Could you check a few things on this model? Use its own coordinates, in mm. A direction names the side the tool comes from. Round coordinates to 2 decimals unless told otherwise and drop trailing zeros. Write each loop counter-clockwise with the first axis right and the second up, starting at its lowest first coordinate (ties: lowest second). Pieces come first, ordered by that corner, then holes. Notation, with made-up numbers: (42.25, 5.5) -> (55.25, 5.5) arc R24 ccw to (55.25, 17.5) -> close; hole circle Ø2 at (62, -8). An arc over 180 degrees is marked (long way). Answer as CSV lines item,"result". Start each with the question number.
Q1. Imagine slicing it at B-B on x = -0.75. Please give me the cut outline in (y, z).
Q2. Imagine slicing it at A-A on z = 30. Please give me the cut outline in (x, y), and give its area (3 significant figures).
Q3. Imagine slicing it at D-D on y = -2.25. Please give me the cut outline in (x, z).
Q4. For faces 4 (the flat face through (-6, -3.355, 11)), 5 (the flat face through (3, 3, 50)), 6 (the flat face through (-2, -6, 41)), which set-ups out of +Z, -Z, +X, -X, +Y, -Y let a thin tool reach every point of the face, with its end or its side?
Q5. If we mould it in two halves opening along Z, with no side actions, what happens to faces 1 (the flat face through (3, 3, -20)), 2 (the flat face through (-3.974, 4.075, 43.535)), 3 (the flat face through (-1, 7.895, 15))? For each: pulls with the +Z half, pulls with the -Z half, needs draft (parallel to the pull), parting line crosses it, or undercut.
Q6. If I drill on line 1 (Z direction, x = -0.75, y = 5.15); line 2 (Y direction, x = -5.75, z = 38.5); line 3 (X direction, y = -1.25, z = 13.5), over which ranges is the centre line in solid material (lowest first)? Write a range as [from, to].
Q7. Will this pin go through, and if not, where does the flat tip stop? pin 1 Ø4 at (x, z) = (-0.75, 30) entering from +Y.
Q8. Imagine slicing it at C-C on z = -7.5. Please give me the cut outline in (x, y).
from build123d import *
from build123d.topology import SkipClean

# Parameters (mm, degrees)
BOSS_EXTRUDE1_START = -20
SKETCH1_W           = 17.5
SKETCH1_H           = 17.5
BOSS_EXTRUDE1_DEPTH = 70
SKETCH2_R           = 4.75
CUT_EXTRUDE1_DEPTH  = 150
SKETCH3_R           = 3.5
CUT_EXTRUDE6_DEPTH  = 25
CUT_EXTRUDE9_START  = -4
CUT_EXTRUDE9_DEPTH  = 66
CUT_EXTRUDE13_START = -4
CUT_EXTRUDE13_DEPTH = 5


with BuildPart() as part:
    # Sketch1 → Boss-Extrude1 (new body)
    with BuildSketch(Plane.XY.offset(BOSS_EXTRUDE1_START)):
        with Locations((-0.75, -0.85483871)):
            Rectangle(SKETCH1_W, SKETCH1_H)
    extrude(amount=BOSS_EXTRUDE1_DEPTH)

    # Sketch2 → Cut-Extrude1 (cut)
    with BuildSketch(Plane(origin=(0, 0, -20), x_dir=(-1, 0, 0), z_dir=(0, 0, -1))):
        with Locations((0.75, -0.85483871)):
            Circle(SKETCH2_R)
    extrude(amount=-CUT_EXTRUDE1_DEPTH, mode=Mode.SUBTRACT)

    # Sketch3 → Cut-Extrude6 (cut)
    with BuildSketch(Plane(origin=(0, 7.89516129, 0), x_dir=(1, 0, 0), z_dir=(0, 1, 0))):
        with Locations(Location((-0.75, -30, 0), (0, 0, 270))):
            Circle(SKETCH3_R)
    extrude(amount=-CUT_EXTRUDE6_DEPTH, mode=Mode.SUBTRACT)

    # Sketch6 → Cut-Extrude9 (cut)
    with BuildSketch(Plane.XY.offset(50).offset(CUT_EXTRUDE9_START)):
        with BuildLine():
            Line((-7.288348415, 1.64516129), (5.788348415, 1.64516129))
            ThreePointArc((5.788348415, 1.64516129), (6.25, -0.85483871), (5.788348415, -3.35483871))
            Line((5.788348415, -3.35483871), (-7.288348415, -3.35483871))
            ThreePointArc((-7.288348415, -3.35483871), (-7.75, -0.85483871), (-7.288348415, 1.64516129))
        make_face()
    extrude(amount=-CUT_EXTRUDE9_DEPTH, mode=Mode.SUBTRACT)

    # Sketch4 → Cut-Extrude13 (cut)
    with SkipClean():  # the faces are left unmerged after this step: merging them gives an invalid solid
        with BuildSketch(Plane.XY.offset(50).offset(CUT_EXTRUDE13_START)):
            with BuildLine():
                ThreePointArc((1.849543844, -4.830372863), (1.468272605, -5.05504902), (1.067746304, -5.243266489))
                Line((1.067746304, -5.243266489), (1.928784027, -7.321995437))
                ThreePointArc((1.928784027, -7.321995437), (2.519033312, -7.044622325), (3.080906718, -6.71352062))
                Line((3.080906718, -6.71352062), (1.849543844, -4.830372863))
            make_face()
            with BuildLine():
                ThreePointArc((1.067746304, -5.243266489), (-3.388958607, -4.804319368), (-5.5, -0.85483871))
                Line((-5.5, -0.85483871), (-7.75, -0.85483871))
                ThreePointArc((-7.75, -0.85483871), (-4.638991631, -6.675125996), (1.928784027, -7.321995437))
                Line((1.928784027, -7.321995437), (1.067746304, -5.243266489))
            make_face()
            with BuildLine():
                ThreePointArc((-3.349543844, 3.120695443), (-2.968272605, 3.345371601), (-2.567746304, 3.53358907))
                Line((-2.567746304, 3.53358907), (-3.428784027, 5.612318018))
                ThreePointArc((-3.428784027, 5.612318018), (-4.019033312, 5.334944906), (-4.580906718, 5.0038432))
                Line((-4.580906718, 5.0038432), (-3.349543844, 3.120695443))
            make_face()
            with BuildLine():
                ThreePointArc((-2.567746304, 3.53358907), (1.888958607, 3.094641949), (4, -0.85483871))
                Line((4, -0.85483871), (6.25, -0.85483871))
                ThreePointArc((6.25, -0.85483871), (3.138991631, 4.965448576), (-3.428784027, 5.612318018))
                Line((-3.428784027, 5.612318018), (-2.567746304, 3.53358907))
            make_face()
        extrude(amount=-CUT_EXTRUDE13_DEPTH, mode=Mode.SUBTRACT)


solid = part.part
Checks:
1,outline,"(-9.6, -20) -> (-5.6, -20) -> (-5.6, 26.5) -> (-9.6, 26.5) -> close; (-9.6, 33.5) -> (-5.6, 33.5) -> (-5.6, 41) -> (-7.85, 41) -> (-7.85, 46) -> (-5.6, 46) -> (-5.6, 50) -> (-9.6, 50) -> close; (3.9, -20) -> (7.9, -20) -> (7.9, 26.5) -> (3.9, 26.5) -> close; (3.9, 33.5) -> (7.9, 33.5) -> (7.9, 50) -> (3.9, 50) -> (3.9, 46) -> (6.15, 46) -> (6.15, 41) -> (3.9, 41) -> close"
2,outline,"(-9.5, -9.6) -> (-4.25, -9.6) -> (-4.25, -4.07) arc R4.75 cw to (-4.79, -3.35) -> (-7.29, -3.35) arc R7 cw to (-7.29, 1.65) -> (-4.79, 1.65) arc R4.75 cw to (-4.25, 2.36) -> (-4.25, 7.9) -> (-9.5, 7.9) -> close; (2.75, -9.6) -> (8, -9.6) -> (8, 7.9) -> (2.75, 7.9) -> (2.75, 2.36) arc R4.75 cw to (3.29, 1.65) -> (5.79, 1.65) arc R7 cw to (5.79, -3.35) -> (3.29, -3.35) arc R4.75 cw to (2.75, -4.07) -> close"
2,area,"149 mm^2"
3,outline,"(-9.5, -20) -> (-7.61, -20) -> (-7.61, 46) -> (-5.29, 46) -> (-5.29, 50) -> (-9.5, 50) -> close; (3.79, 46) -> (6.11, 46) -> (6.11, -20) -> (8, -20) -> (8, 50) -> (3.79, 50) -> close"
4,face 4,"-Z"
4,face 5,"+Z, +X, -X, +Y, -Y"
4,face 6,"none"
5,face 1,"pulls with the -Z half"
5,face 2,"undercut"
5,face 3,"needs draft"
6,line 1,"[-20, 26.5], [33.5, 41], [46, 50]"
6,line 2,"[-9.6, -3.35], [1.65, 7.9]"
6,line 3,"[-9.5, -7.74], [6.24, 8]"
7,pin 1,"through"
8,outline,"(-9.5, -9.6) -> (8, -9.6) -> (8, 7.9) -> (-9.5, 7.9) -> close; hole (-7.29, -3.35) -> (-4.79, -3.35) arc R4.75 ccw to (3.29, -3.35) -> (5.79, -3.35) arc R7 ccw to (5.79, 1.65) -> (3.29, 1.65) arc R4.75 ccw to (-4.79, 1.65) -> (-7.29, 1.65) arc R7 ccw to start"
